from build123d import *

# Parameters (mm, degrees)
F0_R     = 19
F0_R_2   = 14
F0_R_3   = 10
F1_DEPTH = 5
F2_DEPTH = 25
F3_SIZE  = 4.99999
F4_SIZE  = 2
F5_R     = 6.7


# Not quite as in the source:
# - a fillet or chamfer is up to 0.001 mm smaller than in the source, because OpenCascade refuses the exact size


with BuildPart() as f1:
    # F0 (on Front) → F1 (new body)
    with BuildSketch(Plane.XZ):
        Circle(F0_R)
        Circle(F0_R_2, mode=Mode.SUBTRACT)
        Circle(F0_R_2)
        Circle(F0_R_3, mode=Mode.SUBTRACT)
    extrude(amount=F1_DEPTH)

    # F0 (on Front) → F2 (join)
    with BuildSketch(Plane.XZ):
        Circle(F0_R_2)
        Circle(F0_R_3, mode=Mode.SUBTRACT)
    extrude(amount=-F2_DEPTH)

    # F3 (size 5 in the source; OpenCascade refuses exactly that, so slightly less here)
    f3_edges = [f1.edges().sort_by_distance(p)[0] for p in [
        (-19, -5, 0),
    ]]
    chamfer(f3_edges, length=F3_SIZE)

    # F4
    f4_edges = [f1.edges().sort_by_distance(p)[0] for p in [
        (-10, 25, 0),
    ]]
    chamfer(f4_edges, length=F4_SIZE)

    # F5
    f5_edges = [f1.edges().sort_by_distance(p)[0] for p in [
        (-10, 23, 0),
    ]]
    fillet(f5_edges, radius=F5_R)


solid = f1.part
For this review, take the finished solid that the model builds, in its own axes (mm). A direction names the side the tool comes from. Round coordinates to 2 decimals unless told otherwise and drop trailing zeros. Loops run counter-clockwise (first coordinate to the right, second up) from the corner with the lowest first, then second, coordinate; pieces in that order, holes last. Notation, with made-up numbers: (-15, 6) - (19, 6) arc R17 ccw to (19, 30) - close; hole circle Ø8 at (-23.75, 41.25). An arc over 180 degrees is marked (long way). One line per item, written item: value. Start each with the question number.
Item 1: For L1, parallel to Z at x = 0, y = 2; L2, parallel to X at y = 16.5, z = 8; L3, parallel to X at y = 18, z = 7, list the stretches that pass through material, from the lowest coordinate up.
Item 2: Clearance check with flat-ended pins moving along their axes: pin 1 Ø3 at (y, z) = (15.5, 0.5) entering from +X; pin 2 Ø12 at (x, y) = (-6.5, 17) entering from +Z; pin 3 Ø3 at (y, z) = (4, 10) entering from +X; pin 4 Ø16 at (x, z) = (0, 0) entering from +Y. State where each tip first meets the part, or that it passes through.
Item 3: For faces 1 (the flat face through (-6.3, 25, 10.4)), 2 (the cylindrical face through (12.932, 12.325, -5.362)), list the 3-axis set-ups (+Z, -Z, +X, -X, +Y, -Y) from which the entire face can be reached by the end or side of a thin tool; tool diameter is ignored.
Item 4: Take a section at A-A (y = 17). Give the boundary of the cut face in (x, z), plus the area to 3 significant figures.
Item 5: The part is to be moulded in two halves that separate along Z. For faces 3 (the cylindrical face through (5.38, 7.79, 8.43)), 4 (the conical face through (-3.09, -4.76, -13.9)), 5 (the flat face through (-10, -5, 3)), say which applies: +Z half, -Z half, draft (parallel to the pull), parting line (faces both ways), or undercut.
Answer below:
1. L1: z = -14 to -10, 10 to 14
1. L2: x = -11.49 to -6, 6 to 11.49
1. L3: x = -12.12 to -7.14, 7.14 to 12.12
2. pin 1: stops at x = 14
2. pin 2: stops at z = 13.99
2. pin 3: stops at x = 11.12
2. pin 4: passes through
3. face 1: +Z, -Z, +X, -X, +Y
3. face 2: +Y
4. outline: circle Ø28 at (0, 0); hole circle Ø20 at (0, 0)
4. area: 302 mm2
5. face 3: undercut
5. face 4: parting line
5. face 5: draft
